Model file for the job. Use its own axes, mm. Face numbers are marked on the shaded views. A direction names the side the tool comes from. Round coordinates to 2 decimals unless told otherwise and drop trailing zeros. Loops run counter-clockwise (first coordinate to the right, second up) from the corner with the lowest first, then second, coordinate; pieces in that order, holes last. Notation, with made-up numbers: (-39, 65) - (-33, 65) arc R35 cw to (-33, 99) - close; hole circle Ø4 at (43, 69). An arc over 180 degrees is marked (long way). Use one line per item in the form item = value.
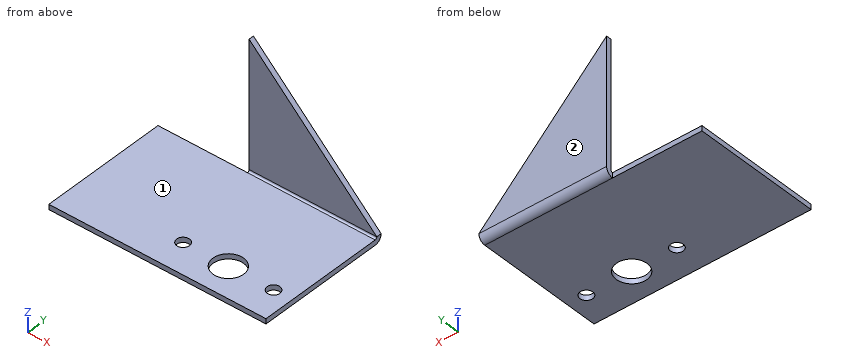
from build123d import *

# Parameters (mm, degrees)
CROQUIS1_W             = 85
CROQUIS1_H             = 50
BRIDA_BASE1_DEPTH      = 2
BRIDA_DE_ARISTA1_DEPTH = 85
DESDOBLAR1_START       = -42.5
DESDOBLAR1_DEPTH       = 85
DESDOBLAR1_2_DEPTH     = 85
CROQUIS11_W            = 35
CROQUIS11_H            = 49.2634
CROQUIS11_H_2          = 2.727844901
CORTAR_EXTRUIR1_DEPTH  = 10
DOBLAR1_START          = 27.727844901
DOBLAR1_OUTLINE_W      = 50
DOBLAR1_OUTLINE_H      = 2
DOBLAR1_DEPTH          = 50.272155099
DOBLAR1_START_2        = 25.7366
DOBLAR1_2_DEPTH        = 1.725934706
DOBLAR1_START_3        = 25
DOBLAR1_3_DEPTH        = 2.7366
DOBLAR1_START_4        = -7.5
DOBLAR1_4_DEPTH        = 50.5
CROQUIS12_R            = 6
CROQUIS12_R_2          = 2.5
CORTAR_EXTRUIR2_DEPTH  = 10


with BuildPart() as part:
    # Brida base1: sheet metal written as solids
    # Croquis1 → Brida base1 (new body)
    with BuildSketch(Plane.XY):
        Rectangle(CROQUIS1_W, CROQUIS1_H)
    extrude(amount=-BRIDA_BASE1_DEPTH)

    # Brida de arista1: sheet metal written as solids
    # Brida de arista1 section (on a plane across the edge) → Brida de arista1 (add)
    with BuildSketch(Plane(origin=(42.5, 25.7366, 0), x_dir=(0, -1, 0), z_dir=(-1, 0, 0))):
        with BuildLine():
            Line((-2, 0.7366), (-2, 50))
            Line((-2, 50), (0, 50))
            Line((0, 50), (0, 0.7366))
            ThreePointArc((0, 0.7366), (0.215745145, 0.215745145), (0.7366, 0))
            Line((0.7366, 0), (0.7366, -2))
            ThreePointArc((0.7366, -2), (-1.198468417, -1.198468417), (-2, 0.7366))
        make_face()
    extrude(amount=BRIDA_DE_ARISTA1_DEPTH)

    # Desdoblar1: read off the stored shape, not the designer's step
    # Desdoblar1 outline → Desdoblar1 (cut)
    with BuildSketch(Plane.YZ.offset(DESDOBLAR1_START)):
        with BuildLine():
            Line((25, 0), (27.635602398, 0))
            ThreePointArc((27.635602398, 0), (27.711233029, 0.364854094), (27.7366, 0.7366))
            Line((27.7366, 0.7366), (27.7366, 50))
            Line((27.7366, 50), (25.7366, 50))
            Line((25.7366, 50), (25.7366, 0.7366))
            ThreePointArc((25.7366, 0.7366), (25.520854855, 0.215745145), (25, 0))
        make_face()
    extrude(amount=DESDOBLAR1_DEPTH, mode=Mode.SUBTRACT)

    # Desdoblar1 2 outline → Desdoblar1 2 (add)
    with BuildSketch(Plane.YZ.offset(DESDOBLAR1_START)):
        with BuildLine():
            Line((25, -2), (76.991244901, -2))
            Line((76.991244901, -2), (76.991244901, 0))
            Line((76.991244901, 0), (27.635602398, 0))
            ThreePointArc((27.635602398, 0), (26.654267209, -1.443395312), (25, -2))
        make_face()
    extrude(amount=DESDOBLAR1_2_DEPTH)

    # Croquis11 → Cortar-Extruir1 (cut)
    with BuildSketch(Plane.XY):
        with Locations((-25, 52.359544901)):
            Rectangle(CROQUIS11_W, CROQUIS11_H)
        with Locations((-25, 26.36392245)):
            Rectangle(CROQUIS11_W, CROQUIS11_H_2)
        Polygon((42.5, 76.991244901), (-7.5, 76.991244901), (42.5, 27.727844901), align=None)
    extrude(amount=-CORTAR_EXTRUIR1_DEPTH, mode=Mode.SUBTRACT)

    # Doblar1: read off the stored shape, not the designer's step
    # Doblar1 outline → Doblar1 (cut)
    with BuildSketch(Plane(origin=(0, 0, 0), x_dir=(1, 0, 0), z_dir=(0, 1, 0)).offset(DOBLAR1_START)):
        with Locations((17.5, 1)):
            Rectangle(DOBLAR1_OUTLINE_W, DOBLAR1_OUTLINE_H)
    extrude(amount=DOBLAR1_DEPTH, mode=Mode.SUBTRACT)

    # Doblar1 2 outline → Doblar1 2 (add)
    with BuildSketch(Plane(origin=(0, 0, 0), x_dir=(1, 0, 0), z_dir=(0, 1, 0)).offset(DOBLAR1_START_2)):
        Polygon((-7.5, -50), (42.5, -0.7366), (42.5, 0), (-7.5, 0), align=None)
    extrude(amount=DOBLAR1_2_DEPTH)

    # Doblar1 3 outline → Doblar1 3 (add)
    with BuildSketch(Plane(origin=(0, 0, 0), x_dir=(1, 0, 0), z_dir=(0, 1, 0)).offset(DOBLAR1_START_3)):
        Polygon((-7.5, 0), (-7.5, -50), (42.5, -0.7366), (42.5, 0), align=None)
    extrude(amount=DOBLAR1_3_DEPTH)

    # Doblar1 4 outline → Doblar1 4 (cut)
    with BuildSketch(Plane.YZ.offset(DOBLAR1_START_4)):
        with BuildLine():
            ThreePointArc((27.7366, 0.7366), (26.935068417, -1.198468417), (25, -2))
            Line((25, -2), (24, -2))
            Line((24, -2), (24, -4))
            Line((24, -4), (27.727844901, -4))
            Line((27.727844901, -4), (27.727844901, 0))
            Line((27.727844901, 0), (29, 0))
            Line((29, 0), (29, 52))
            Line((29, 52), (27.736600025, 52))
            Line((27.736600025, 52), (27.7366, 0.7366))
        make_face()
        with BuildLine():
            Line((25.7366, 0.7366), (25.7366, 52))
            Line((25.7366, 52), (25, 52))
            Line((25, 52), (25, 0))
            ThreePointArc((25, 0), (25.520854855, 0.215745145), (25.7366, 0.7366))
        make_face()
    extrude(amount=DOBLAR1_4_DEPTH, mode=Mode.SUBTRACT)

    # Croquis12 → Cortar-Extruir2 (cut)
    with BuildSketch(Plane.XY):
        with Locations((17.5, -13)):
            Circle(CROQUIS12_R)
        with Locations((35.2, -13)):
            Circle(CROQUIS12_R_2)
        with Locations((-0.2, -13)):
            Circle(CROQUIS12_R_2)
    extrude(amount=-CORTAR_EXTRUIR2_DEPTH, mode=Mode.SUBTRACT)


solid = part.part
1. Cut at B-B, the plane x = 35.2. Give the cut face in (y, z), plus the area to 3 significant figures.
Geometry check:
outline = (-25, -2) - (-15.5, -2) - (-15.5, 0) - (-25, 0) - close; (-10.5, -2) - (25, -2) arc R2.74 ccw to (27.74, 0.74) - (27.74, 7.93) - (25.74, 7.93) - (25.74, 0.74) arc R0.74 cw to (25, 0) - (-10.5, 0) - close
area = 110 mm^2
2. Cut at C-C, the plane x = -24.5. Give the cut face in (y, z).
Geometry check:
outline = (-25, -2) - (25, -2) - (25, 0) - (-25, 0) - close
3. Flat gauge pins, fed straight in: pin 1 (12 mm diameter, centred on x = 2, z = 36.5, fed in from -Y); pin 2 (6 mm diameter, centred on x = -0.2, y = -13, fed in from +Z); pin 3 (0.8 mm diameter, centred on y = 26, z = 14, fed in from -X). Where does each tip first touch, or does it go through?
Geometry check:
pin_1 = 25.74
pin_2 = 0
pin_3 = -7.5
4. Cut at A-A, the plane y = -13. Give the cut face in (x, z), plus the area to 3 significant figures.
Geometry check:
outline = (-42.5, -2) - (-2.7, -2) - (-2.7, 0) - (-42.5, 0) - close; (2.3, -2) - (11.5, -2) - (11.5, 0) - (2.3, 0) - close; (23.5, -2) - (32.7, -2) - (32.7, 0) - (23.5, 0) - close; (37.7, -2) - (42.5, -2) - (42.5, 0) - (37.7, 0) - close
area = 126 mm^2
5. Tool access for the marked faces 1 and 2: list every direction of +Z, -Z, +X, -X, +Y, -Y with a clear straight run to the whole face (end or side of a thin tool).
Geometry check:
face_1 = +Z, +X, -X, -Y
face_2 = +Z, -Z, +X, -X, +Y
6. Wall check: probe 1 along Z at (x, y) = (-30.5, -7); probe 2 along Y at (x, z) = (10, 22); probe 3 along Y at (x, z) = (0, -1) (3 decimals). Give the ranges that are in metal, low to high.
Geometry check:
probe_1 = -2 to 0
probe_2 = 25.74 to 27.74
probe_3 = -25 to -15.492, -10.508 to 27.115
7. Cut at D-D, the plane y = 5. Give the cut face in (x, z), plus the area to 3 significant figures.
Geometry check:
outline = (-42.5, -2) - (42.5, -2) - (42.5, 0) - (-42.5, 0) - close
area = 170 mm^2
